```python
from build123d import *

# Parameters (mm, degrees)
BOSS_EXTRUDE1_DEPTH = 15
SKETCH2_R           = 2.25
CUT_EXTRUDE1_DEPTH  = 30.849623113
CUT_EXTRUDE2_START  = -15
CUT_EXTRUDE2_DEPTH  = 15
CUT_EXTRUDE3_DEPTH  = 12.25
CUT_EXTRUDE4_DEPTH  = 11
SKETCH8_W           = 5
SKETCH8_H           = 7
CUT_EXTRUDE5_DEPTH  = 8


with BuildPart() as part:
    # Sketch1 → Boss-Extrude1 (new, symmetric)
    with BuildSketch(Plane.XY):
        with BuildLine():
            Line((15, 0), (-15, 0))
            Line((-15, 0), (-15, -21))
            Line((-15, -21), (-5, -21))
            Line((-5, -21), (-5, -14))
            ThreePointArc((-5, -14), (0, -9), (5, -14))
            Line((5, -14), (5, -21))
            Line((5, -21), (15, -21))
            Line((15, -21), (15, 0))
        make_face()
    extrude(amount=BOSS_EXTRUDE1_DEPTH, both=True)

    # Sketch2 → Cut-Extrude1 (cut, through all)
    with BuildSketch(Plane(origin=(0, 0, 0), x_dir=(1, 0, 0), z_dir=(0, 1, 0))):
        with Locations(Location((-10, 9, 0), (0, 0, 270))):
            Circle(SKETCH2_R)
        with Locations(Location((10, 9, 0), (0, 0, 270))):
            Circle(SKETCH2_R)
        with Locations(Location((10, -9, 0), (0, 0, 270))):
            Circle(SKETCH2_R)
        with Locations(Location((-10, -9, 0), (0, 0, 270))):
            Circle(SKETCH2_R)
    extrude(amount=-CUT_EXTRUDE1_DEPTH, mode=Mode.SUBTRACT)

    # Sketch3 → Cut-Extrude2 (cut)
    with BuildSketch(Plane.XZ.offset(21).offset(CUT_EXTRUDE2_START)):
        with BuildLine():
            Line((-10, 11.25), (10, 11.25))
            ThreePointArc((10, 11.25), (12.25, 9), (10, 6.75))
            Line((10, 6.75), (-10, 6.75))
            ThreePointArc((-10, 6.75), (-12.25, 9), (-10, 11.25))
        make_face()
        with BuildLine():
            Line((10, -11.25), (-10, -11.25))
            ThreePointArc((-10, -11.25), (-12.25, -9), (-10, -6.75))
            Line((-10, -6.75), (10, -6.75))
            ThreePointArc((10, -6.75), (12.25, -9), (10, -11.25))
        make_face()
    extrude(amount=CUT_EXTRUDE2_DEPTH, mode=Mode.SUBTRACT)

    # Sketch4 → Cut-Extrude3 (cut, symmetric)
    with BuildSketch(Plane.XY):
        with BuildLine():
            Line((-7.5, -14), (-7.5, -21))
            Line((-7.5, -21), (7.5, -21))
            Line((7.5, -21), (7.5, -14))
            ThreePointArc((7.5, -14), (0, -6.5), (-7.5, -14))
        make_face()
    extrude(amount=CUT_EXTRUDE3_DEPTH, both=True, mode=Mode.SUBTRACT)

    # Sketch7 → Cut-Extrude4 (cut)
    with BuildSketch(Plane(origin=(15, 0, 0), x_dir=(0, 0, -1), z_dir=(1, 0, 0))):
        with BuildLine():
            Line((-1.590990258, -4.590990258), (0, -6.181980515))
            Line((0, -6.181980515), (1.590990258, -4.590990258))
            ThreePointArc((1.590990258, -4.590990258), (0, -0.75), (-1.590990258, -4.590990258))
        make_face()
    extrude(amount=-CUT_EXTRUDE4_DEPTH, mode=Mode.SUBTRACT)

    # Sketch8 → Cut-Extrude5 (cut)
    with BuildSketch(Plane(origin=(0, 0, 0), x_dir=(1, 0, 0), z_dir=(0, 1, 0))):
        with Locations((8.5, 0)):
            Rectangle(SKETCH8_W, SKETCH8_H)
    extrude(amount=-CUT_EXTRUDE5_DEPTH, mode=Mode.SUBTRACT)


solid = part.part
```
CAD build for the part. Positions are in the model's coordinates, mm. A direction names the side the tool comes from. Round coordinates to 2 decimals unless told otherwise and drop trailing zeros. Order: outer loops, then holes, each group sorted by start corner. A loop starts at its lowest first (then second) coordinate and runs counter-clockwise, first axis right, second up.
Q1. Two-plate mould, pull along Z, no slides. Class faces 1 (the flat face through (0, -6.2, 6.75)), 2 (the flat face through (0, 0, 0)), 3 (the flat face through (0, -8, 15)), 4 (the flat face through (-7.5, -17, -12)): pulls with the +Z half, pulls with the -Z half, needs draft (parallel to the pull), parting line crosses it, or undercut.
Q2. Wall check: L1, parallel to Z at x = -9.75, y = -8.5; L2, parallel to X at y = -5.75, z = -9; L3, parallel to Z at x = 10, y = -4.75. Give the ranges that are in metal, low to high.
Q3. Which spindle directions (+Z, -Z, +X, -X, +Y, -Y) get a long thin tool onto all of the face, cutting with end or side? Do faces 5 (the flat face through (5.014, -5.375, 0.807)), 6 (the flat face through (6, -5, -2)), 7 (the flat face through (-0.1, -8.8, 12.25)). Say none if no direction does.
Q4. Slice it at D-D (x = -6). Write the cut outline in (y, z).
Q5. Slice it at B-B (z = -9). Write the cut outline in (x, y).
Q6. Drop flat-ended pins along their axis: pin 1 (1.3 mm diameter, centred on x = 2, z = -8, fed in from -Y); pin 2 (2 mm diameter, centred on y = -2.5, z = 1, fed in from +X). Give the stop position or say it passes through.
Q7. Slice it at C-C (y = -3). Write the cut outline in (x, z), and give its area (3 significant figures).
Results below:
1. face 1: undercut
1. face 2: needs draft
1. face 3: pulls with the +Z half
1. face 4: undercut
2. L1: z = -15 to -11.25, -6.75 to 6.75, 11.25 to 15
2. L2: x = -15 to -12.25, -7.75 to 7.75, 12.25 to 15
2. L3: z = -15 to -11.25, -6.75 to -3.5, 3.5 to 6.75, 11.25 to 15
3. face 5: +X
3. face 6: +Y
3. face 7: -Y
4. outline: (-21, -15) - (0, -15) - (0, 15) - (-21, 15) - (-21, 12.25) - (-9.5, 12.25) - (-9.5, 11.25) - (-6, 11.25) - (-6, 6.75) - (-9.5, 6.75) - (-9.5, -6.75) - (-6, -6.75) - (-6, -11.25) - (-9.5, -11.25) - (-9.5, -12.25) - (-21, -12.25) - close
5. outline: (-15, -21) - (-12.25, -21) - (-12.25, 0) - (-15, 0) - close; (-7.75, -6) - (7.75, -6) - (7.75, 0) - (-7.75, 0) - close; (12.25, -21) - (15, -21) - (15, 0) - (12.25, 0) - close
6. pin 1: stops at y = -6
6. pin 2: stops at x = 4
7. outline: (-15, -15) - (15, -15) - (15, -2.25) - (11, -2.25) - (11, -3.5) - (6, -3.5) - (6, -2.25) - (4, -2.25) - (4, 2.25) - (6, 2.25) - (6, 3.5) - (11, 3.5) - (11, 2.25) - (15, 2.25) - (15, 15) - (-15, 15) - close; hole circle Ø4.5 at (-10, -9); hole circle Ø4.5 at (-10, 9); hole circle Ø4.5 at (10, -9); hole circle Ø4.5 at (10, 9)
7. area: 774 mm2
